Geometry check sheet. Reference: the model listing, model coordinates, mm. Round coordinates to 2 decimals unless told otherwise and drop trailing zeros. Write each loop counter-clockwise with the first axis right and the second up, starting at its lowest first coordinate (ties: lowest second). Pieces come first, ordered by that corner, then holes.
from build123d import *

# Parameters (mm, degrees)
F1_DEPTH = 25


with BuildPart() as f1:
    # F0 (on Top) → F1 (new body)
    with BuildSketch(Plane.XY):
        with BuildLine():
            ThreePointArc((2.9746431824, -0.3892273592), (2.9936540838, -0.1950262196), (3, 0))
            ThreePointArc((3, 0), (2.9936540838, 0.1950262196), (2.9746431824, 0.3892273592))
            ThreePointArc((2.9746431824, 0.3892273592), (1.8618249989, 1.8724282704), (0.0077205477, 1.8957935577))
            ThreePointArc((0.0077205477, 1.8957935577), (0.8802141699, 1.1209485987), (1.2044117487, 0))
            ThreePointArc((1.2044117487, 0), (0.8802141699, -1.1209485987), (0.0077205477, -1.8957935577))
            ThreePointArc((0.0077205477, -1.8957935577), (1.8618249989, -1.8724282704), (2.9746431824, -0.3892273592))
        make_face()
        with BuildLine():
            ThreePointArc((0.0077205477, -1.8957935577), (-1.1889706532, 0), (0.0077205477, 1.8957935577))
            ThreePointArc((0.0077205477, 1.8957935577), (-2.9955882513, 0), (0.0077205477, -1.8957935577))
        make_face()
        with BuildLine():
            ThreePointArc((1.2044117487, 0), (0.8802141699, 1.1209485987), (0.0077205477, 1.8957935577))
            ThreePointArc((0.0077205477, 1.8957935577), (-1.1889706532, 0), (0.0077205477, -1.8957935577))
            ThreePointArc((0.0077205477, -1.8957935577), (0.8802141699, -1.1209485987), (1.2044117487, 0))
        make_face()
    extrude(amount=F1_DEPTH)


solid = f1.part
1. Scan lines: line 1 along Y through (x, z) = (-1.05, 22); line 2 along Y through (x, z) = (0.15, 14.75); line 3 along X through (y, z) = (0.7, 10.25). Record each from-to range of solid material in increasing order.
2. Release check for a two-part mould opening along X. For faces 1 (the face through (1.89, 1.86, 12.32)), 2 (the face through (1.838, -1.884, 12.325)), 3 (the face through (0, 0, 0)) record: +X half, -X half, draft (parallel to the pull), parting line (faces both ways), or undercut.
3. Section check A-A (z = 13). Record the cut outline in (x, y), plus the area to 3 significant figures.
4. Depth check by flat-ended pin: pin 1 Ø2 at (x, z) = (2, 20) entering from +Y; pin 2 Ø1 at (x, y) = (2, 0) entering from -Z. Enter the tip coordinate at first touch or a pass-through.
5. Section check B-B (y = -1.3). Record the cut outline in (x, z), plus the area to 3 significant figures.
6. Section check C-C (x = -1.85). Record the cut outline in (y, z).
Results below:
1. line 1: y = -2.09 to 2.09
1. line 2: y = -1.96 to 1.96
1. line 3: x = -2.88 to 2.89
2. face 1: undercut
2. face 2: undercut
2. face 3: draft
3. outline: (0.01, -1.9) arc R2.1 ccw to (2.97, -0.39) arc R3 ccw to (2.97, 0.39) arc R2.1 ccw to (0.01, 1.9) arc R2.1 ccw (long way) to start
3. area: 21.2 mm2
4. pin 1: stops at y = 2.1
4. pin 2: stops at z = 0
5. outline: (-2.54, 0) - (2.56, 0) - (2.56, 25) - (-2.54, 25) - close
5. area: 128 mm2
6. outline: (-1.87, 0) - (1.87, 0) - (1.87, 25) - (-1.87, 25) - close
